Job drawing, mm, ordinate dimensions from the low corner. One solid piece. A direction names the side the tool comes from. Round coordinates to 2 decimals unless told otherwise and drop trailing zeros. Loops run counter-clockwise (first coordinate to the right, second up) from the corner with the lowest first, then second, coordinate; pieces in that order, holes last.
1) 3-axis set-ups, long thin cutter, end or side, ignore diameter. For the marked faces 1 and 2: which of +Z, -Z, +X, -X, +Y, -Y reach the whole face in a straight line?
2) Band-saw the part on B-B, the plane x = 3.5. Write the cut outline in (y, z), then the cut area to 3 significant figures.
3) Band-saw the part on A-A, the plane y = 20. Write the cut outline in (x, z), then the cut area to 3 significant figures.
4) Probe line 1 (X direction, y = 20, z = 4.5); line 2 (Y direction, x = 52.5, z = 8.75); line 3 (Z direction, x = 30, y = 22). List the from-to ranges inside material, lowest first.
5) Drop flat-ended pins along their axis: P1, Ø0.5, axis at y = 20.5, z = 10.5, coming from the -X side; P2, Ø0.5, axis at x = 20, z = 10.5, coming from the +Y side; P3, Ø1, axis at x = 32, y = 18.5, coming from the +Z side. Give the stop position or say it passes through.
6) Band-saw the part on C-C, the plane x = 14. Write the cut outline in (y, z).
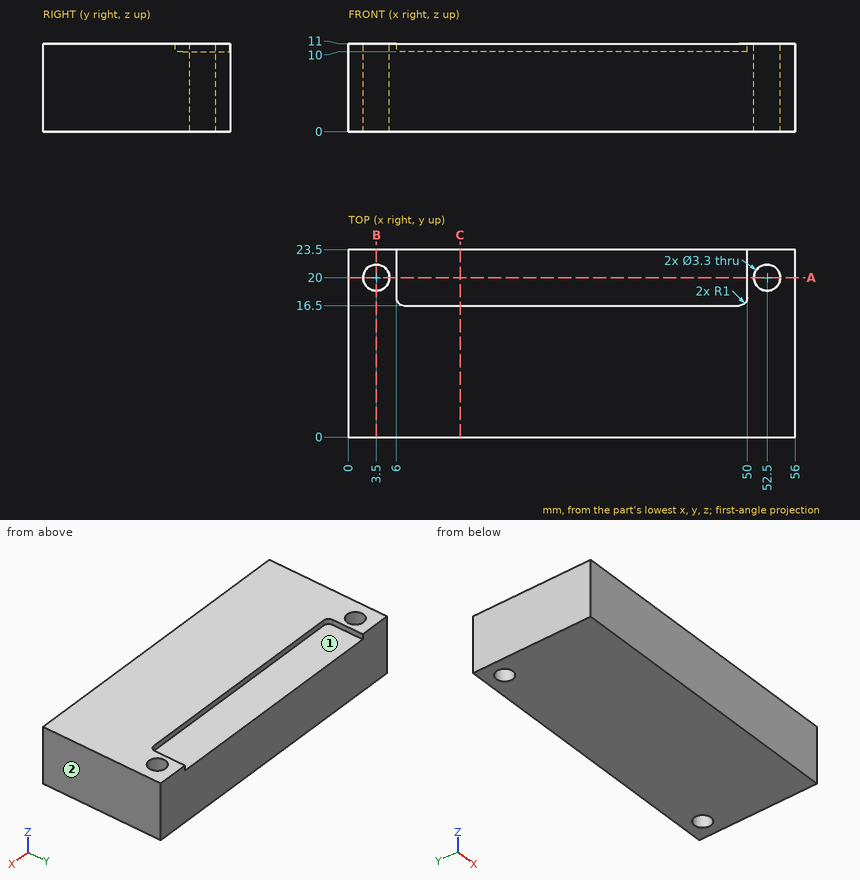
Reported:
1. face 1: +Z, +Y
1. face 2: +Z, -Z, +X, +Y, -Y
2. outline: (0, 0) - (18.35, 0) - (18.35, 11) - (0, 11) - close; (21.65, 0) - (23.5, 0) - (23.5, 11) - (21.65, 11) - close
2. area: 222 mm2
3. outline: (0, 0) - (1.85, 0) - (1.85, 11) - (0, 11) - close; (5.15, 0) - (50.85, 0) - (50.85, 11) - (50, 11) - (50, 10) - (6, 10) - (6, 11) - (5.15, 11) - close; (54.15, 0) - (56, 0) - (56, 11) - (54.15, 11) - close
3. area: 499 mm2
4. line 1: x = 0 to 1.85, 5.15 to 50.85, 54.15 to 56
4. line 2: y = 0 to 18.35, 21.65 to 23.5
4. line 3: z = 0 to 10
5. P1: stops at x = 0
5. P2: stops at y = 16.5
5. P3: stops at z = 10
6. outline: (0, 0) - (23.5, 0) - (23.5, 10) - (16.5, 10) - (16.5, 11) - (0, 11) - close
